from build123d import *

# Parameters (mm, degrees)
SKETCH1_W           = 127
SKETCH1_H           = 127
BOSS_EXTRUDE1_DEPTH = 179
SKETCH2_R           = 25
BOSS_EXTRUDE2_DEPTH = 31.1
SKETCH3_R           = 34.925
BOSS_EXTRUDE3_DEPTH = 15
SKETCH4_R           = 17.5
BOSS_EXTRUDE4_DEPTH = 146


with BuildPart() as part:
    # Sketch1 → Boss-Extrude1 (new body)
    with BuildSketch(Plane.XY):
        Rectangle(SKETCH1_W, SKETCH1_H)
    extrude(amount=BOSS_EXTRUDE1_DEPTH)

    # Sketch2 → Boss-Extrude2 (add)
    with BuildSketch(Plane.XY.offset(179)):
        Circle(SKETCH2_R)
    extrude(amount=BOSS_EXTRUDE2_DEPTH)

    # Sketch3 → Boss-Extrude3 (add)
    with BuildSketch(Plane.XY.offset(210.1)):
        Circle(SKETCH3_R)
    extrude(amount=BOSS_EXTRUDE3_DEPTH)

    # Sketch4 → Boss-Extrude4 (add)
    with BuildSketch(Plane.XY.offset(225.1)):
        Circle(SKETCH4_R)
    extrude(amount=BOSS_EXTRUDE4_DEPTH)


solid = part.part
Here's how the part is built. I have some questions about the finished solid (model axes, mm). A direction names the side the tool comes from. Coordinates: 2 decimals unless noted, no trailing zeros. Loops run counter-clockwise (first coordinate to the right, second up) from the corner with the lowest first, then second, coordinate; pieces in that order, holes last.
1. Imagine slicing it at D-D, the plane z = 272.5. Please give me the cut outline in (x, y), and give its area (3 significant figures).
2. If we mould it in two halves opening along Z, with no side actions, what happens to faces 1 (the flat face through (63.5, -1, 88)), 2 (the flat face through (-16, 8, 225.1)), 3 (the cylindrical face through (23.846, 7.509, 194.332)), 4 (the flat face through (-1, 1, 0))? For each: pulls with the +Z half, pulls with the -Z half, needs draft (parallel to the pull), parting line crosses it, or undercut.
3. I need wall thicknesses on L1, parallel to Z at x = -27.5, y = -8; L2, parallel to Z at x = 24, y = 1; L3, parallel to Z at x = 35, y = 36. Which ranges of each line are inside material? Lowest first, please.
4. For P1, Ø3, axis at x = -5.5, z = 225, coming from the -Y side; P2, Ø10, axis at x = -32, y = -50.5, coming from the -Z side, each with a flat end and sliding along its axis, tell me the tip position at first contact or that it passes through.
5. For faces 5 (the flat face through (-8, 24, 210.1)), 6 (the cylindrical face through (-13.887, -10.648, 297.078)), 7 (the flat face through (-1, -63.5, 88)), which set-ups out of +Z, -Z, +X, -X, +Y, -Y let a thin tool reach every point of the face, with its end or its side?
6. Imagine slicing it at C-C, the plane x = -28.5. Please give me the cut outline in (y, z).
7. Imagine slicing it at A-A, the plane x = 0. Please give me the cut outline in (y, z) (3 decimals), and give its area (3 significant figures).
Taken from the geometry:
1. outline: circle Ø35 at (0, 0)
1. area: 962 mm2
2. face 1: needs draft
2. face 2: pulls with the +Z half
2. face 3: undercut
2. face 4: pulls with the -Z half
3. L1: z = 0 to 179, 210.1 to 225.1
3. L2: z = 0 to 225.1
3. L3: z = 0 to 179
4. P1: stops at y = -34.7
4. P2: stops at z = 0
5. face 5: none
5. face 6: +Z
5. face 7: +Z, -Z, +X, -X, -Y
6. outline: (-63.5, 0) - (63.5, 0) - (63.5, 179) - (-63.5, 179) - close; (-20.19, 210.1) - (20.19, 210.1) - (20.19, 225.1) - (-20.19, 225.1) - close
7. outline: (-63.5, 0) - (63.5, 0) - (63.5, 179) - (25, 179) - (25, 210.1) - (34.925, 210.1) - (34.925, 225.1) - (17.5, 225.1) - (17.5, 371.1) - (-17.5, 371.1) - (-17.5, 225.1) - (-34.925, 225.1) - (-34.925, 210.1) - (-25, 210.1) - (-25, 179) - (-63.5, 179) - close
7. area: 30,400 mm2
